Model file for the job. Use its own axes, mm. A direction names the side the tool comes from. Coordinates: 2 decimals unless noted, no trailing zeros. Order: outer loops, then holes, each group sorted by start corner. A loop starts at its lowest first (then second) coordinate and runs counter-clockwise, first axis right, second up. Notation, with made-up numbers: (72.25, 25.25) - (78.25, 25.25) arc R23 ccw to (78.25, 42.25) - close; hole circle Ø3 at (-19, 13.25). An arc over 180 degrees is marked (long way). Put each result on its own line as item: value. Start each with the question number.
```python
from build123d import *

# Parameters (mm, degrees)
SKETCH1_R           = 6
SKETCH1_R_2         = 1.5
SKETCH1_R_3         = 2
BOSS_EXTRUDE1_DEPTH = 2.5
FILLET1_R           = 25
FILLET2_R           = 10


with BuildPart() as part:
    # Sketch1 → Boss-Extrude1 (new, symmetric)
    with BuildSketch(Plane(origin=(0, 0, 0), x_dir=(1, 0, 0), z_dir=(0, 1, 0))):
        with BuildLine():
            Line((-79, 94), (79, 94))
            ThreePointArc((79, 94), (89.606601718, 89.606601718), (94, 79))
            Line((94, 79), (94, -79))
            ThreePointArc((94, -79), (89.606601718, -89.606601718), (79, -94))
            Line((79, -94), (-79, -94))
            ThreePointArc((-79, -94), (-89.606601718, -89.606601718), (-94, -79))
            Line((-94, -79), (-94, -30))
            Line((-94, -30), (-154, -30))
            Line((-154, -30), (-154, 30))
            Line((-154, 30), (-94, 30))
            Line((-94, 30), (-94, 79))
            ThreePointArc((-94, 79), (-89.606601718, 89.606601718), (-79, 94))
        make_face()
        with Locations(Location((-76.013978978, 76.013978978, 0), (0, 0, 270))):
            Circle(SKETCH1_R, mode=Mode.SUBTRACT)
        with Locations(Location((76.013978978, 76.013978978, 0), (0, 0, 270))):
            Circle(SKETCH1_R, mode=Mode.SUBTRACT)
        with Locations(Location((76.013978978, -76.013978978, 0), (0, 0, 270))):
            Circle(SKETCH1_R, mode=Mode.SUBTRACT)
        with Locations(Location((-76.013978978, -76.013978978, 0), (0, 0, 270))):
            Circle(SKETCH1_R, mode=Mode.SUBTRACT)
        with Locations(Location((-135, -10, 0), (0, 0, 270))):
            Circle(SKETCH1_R_2, mode=Mode.SUBTRACT)
        with Locations(Location((-145, 0, 0), (0, 0, 270))):
            Circle(SKETCH1_R_2, mode=Mode.SUBTRACT)
        with Locations(Location((-135, 10, 0), (0, 0, 270))):
            Circle(SKETCH1_R_2, mode=Mode.SUBTRACT)
        with Locations(Location((-125, 0, 0), (0, 0, 270))):
            Circle(SKETCH1_R_2, mode=Mode.SUBTRACT)
        with Locations(Location((-135, 0, 0), (0, 0, 270))):
            Circle(SKETCH1_R, mode=Mode.SUBTRACT)
        with Locations(Location((13.609798459, 85.928885632, 0), (0, 0, 270))):
            Circle(SKETCH1_R_3, mode=Mode.SUBTRACT)
        with Locations(Location((13.609798458, -85.928885632, 0), (0, 0, 270))):
            Circle(SKETCH1_R_3, mode=Mode.SUBTRACT)
        with Locations(Location((-13.609798458, 85.928885632, 0), (0, 0, 270))):
            Circle(SKETCH1_R_3, mode=Mode.SUBTRACT)
        with Locations(Location((-13.609798459, -85.928885632, 0), (0, 0, 270))):
            Circle(SKETCH1_R_3, mode=Mode.SUBTRACT)
    extrude(amount=BOSS_EXTRUDE1_DEPTH, both=True)

    # Fillet1
    fillet1_edges = [part.edges().sort_by_distance(p)[0] for p in [
        (-94, 0, 30),
        (-94, 0, -30),
    ]]
    fillet(fillet1_edges, radius=FILLET1_R)

    # Fillet2
    fillet2_edges = [part.edges().sort_by_distance(p)[0] for p in [
        (-154, 0, 30),
        (-154, 0, -30),
    ]]
    fillet(fillet2_edges, radius=FILLET2_R)


solid = part.part
```
Item 1: Slice it at A-A, the plane y = 0. Give the number of separate pieces and of enclosed holes in the cut face, plus the area to 3 significant figures.
Item 2: Slice it at B-B, the plane x = -112. Give the cut face in (y, z).
Item 3: Flat gauge pins, fed straight in: pin 1 Ø19 at (x, z) = (-76.01, 76.01) entering from -Y; pin 2 Ø11 at (x, z) = (-135, 0) entering from +Y; pin 3 Ø1.5 at (x, y) = (-127.5, 0.5) entering from +Z; pin 4 Ø2.5 at (y, z) = (-1, 63) entering from -X. Where does each tip first touch, or does it go through?
Item 4: Wall check: line 1 along X through (y, z) = (0.9, 0); line 2 along Z through (x, y) = (-76.5, -0.9); line 3 along X through (y, z) = (-1.9, 78). Give the ranges that are in metal, low to high.
Item 5: Slice it at C-C, the plane z = 32.5. Give the cut face in (x, y), plus the area to 3 significant figures.
Item 6: 3-axis set-ups, long thin cutter, end or side, ignore diameter. For faces 1 (the face through (-1, 2.5, -1)), 2 (the face through (-94, 0, 67)), 3 (the face through (-132, 0, -30)): which of +Z, -Z, +X, -X, +Y, -Y reach the whole face in a straight line?
Item 7: Pull direction Z, two halves, no side cores. Call faces 4 (the face through (-150.99, 0.04, -27.15)), 5 (the face through (77.816, -0.035, -70.291)), 6 (the face through (94, 0, -1)), 7 (the face through (-131, 0, 30)): pulls with the +Z half, pulls with the -Z half, needs draft (parallel to the pull), parting line crosses it, or undercut.
Here are the results:
1. separate pieces: 1
1. enclosed holes: 13
1. area: 38,300 mm^2
2. outline: (-2.5, -31) - (2.5, -31) - (2.5, 31) - (-2.5, 31) - close
3. pin 1: stops at y = -2.5
3. pin 2: passes through
3. pin 3: stops at z = 30
3. pin 4: stops at x = -94
4. line 1: x = -154 to -146.5, -143.5 to -141, -129 to -126.5, -123.5 to 94
4. line 2: z = -94 to -81.99, -70.03 to 70.03, 81.99 to 94
4. line 3: x = -94 to -81.68, -70.35 to 70.35, 81.68 to 94
5. outline: (-108.1, -2.5) - (94, -2.5) - (94, 2.5) - (-108.1, 2.5) - close
5. area: 1,010 mm^2
6. face 1: +Z, -Z, +X, -X, +Y
6. face 2: +Z, -X, +Y, -Y
6. face 3: -Z, -X, +Y, -Y
7. face 4: pulls with the -Z half
7. face 5: undercut
7. face 6: needs draft
7. face 7: pulls with the +Z half
